The listing builds one solid part. Answer for the finished solid, in the listing's coordinates (mm). Face numbers are marked on the shaded views. A direction names the side the tool comes from. Coordinates: 2 decimals unless noted, no trailing zeros. Order: outer loops, then holes, each group sorted by start corner. A loop starts at its lowest first (then second) coordinate and runs counter-clockwise, first axis right, second up. Notation, with made-up numbers: (-20, 82.5) -> (33, 82.5) arc R18 cw to (33, 100.5) -> close; hole circle Ø11 at (72, 85). An arc over 180 degrees is marked (long way). Return JSON: item names as keys, results as strings.
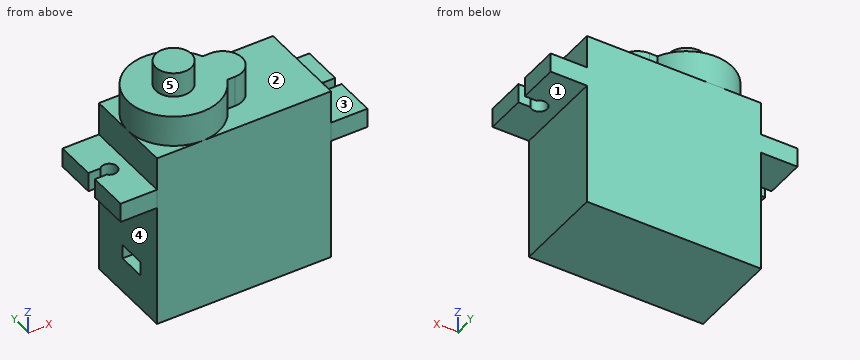
from build123d import *

# Parameters (mm, degrees)
CROQUIS1_W              = 22.5
CROQUIS1_H              = 11.8
SALIENTE_EXTRUIR1_DEPTH = 22.7
SALIENTE_EXTRUIR2_DEPTH = 2.5
SALIENTE_EXTRUIR3_DEPTH = 4
CROQUIS4_R              = 2.3
SALIENTE_EXTRUIR4_DEPTH = 3.2
CROQUIS5_W              = 1.844144091
CROQUIS5_H              = 3.6
CORTAR_EXTRUIR1_DEPTH   = 1.6


with BuildPart() as part:
    # Croquis1 → Saliente-Extruir1 (new body)
    with BuildSketch(Plane.XY):
        Rectangle(CROQUIS1_W, CROQUIS1_H)
    extrude(amount=SALIENTE_EXTRUIR1_DEPTH)

    # Croquis2 → Saliente-Extruir2 (add)
    with BuildSketch(Plane.XY.offset(15.9)):
        with BuildLine():
            Line((11.25, 5.9), (15.95, 5.9))
            Line((15.95, 5.9), (15.95, 0.647985587))
            Line((15.95, 0.647985587), (14.411652597, 0.647985587))
            ThreePointArc((14.411652597, 0.647985587), (12.650003513, 0.00265078), (14.408206572, -0.652014413))
            Line((14.408206572, -0.652014413), (15.95, -0.652014413))
            Line((15.95, -0.652014413), (15.95, -5.904028826))
            Line((15.95, -5.904028826), (11.25, -5.904028826))
            Line((11.25, -5.904028826), (11.25, 5.9))
        make_face()
        with BuildLine():
            Line((-11.25, 5.9), (-15.95, 5.9))
            Line((-15.95, 5.9), (-15.95, 0.647985587))
            Line((-15.95, 0.647985587), (-14.411652597, 0.647985587))
            ThreePointArc((-14.411652597, 0.647985587), (-12.650003513, 0.00265078), (-14.408206572, -0.652014413))
            Line((-14.408206572, -0.652014413), (-15.95, -0.652014413))
            Line((-15.95, -0.652014413), (-15.95, -5.904028826))
            Line((-15.95, -5.904028826), (-11.25, -5.904028826))
            Line((-11.25, -5.904028826), (-11.25, 5.9))
        make_face()
    extrude(amount=SALIENTE_EXTRUIR2_DEPTH)

    # Croquis3 → Saliente-Extruir3 (add)
    with BuildSketch(Plane.XY.offset(22.7)):
        with BuildLine():
            Line((1.003159638, -2.50231492), (-0.006927846, -2.50231492))
            ThreePointArc((-0.006927846, -2.50231492), (-11.24999987, 0.001237918), (-0.005878262, 2.500072568))
            Line((-0.005878262, 2.500072568), (1.003159638, 2.500072568))
            ThreePointArc((1.003159638, 2.500072568), (3.504353382, -0.001121176), (1.003159638, -2.50231492))
        make_face()
    extrude(amount=SALIENTE_EXTRUIR3_DEPTH)

    # Croquis4 → Saliente-Extruir4 (add)
    with BuildSketch(Plane.XY.offset(26.7)):
        with Locations((-5.35, 0)):
            Circle(CROQUIS4_R)
    extrude(amount=SALIENTE_EXTRUIR4_DEPTH)

    # Croquis5 → Cortar-Extruir1 (cut, symmetric)
    with BuildSketch(Plane.ZY.offset(11.25)):
        with Locations((5.422072046, -0.7)):
            Rectangle(CROQUIS5_W, CROQUIS5_H)
    extrude(amount=CORTAR_EXTRUIR1_DEPTH, both=True, mode=Mode.SUBTRACT)


solid = part.part
1. Consider line 1 (Y direction, x = -13.65, z = 17.4); line 2 (Y direction, x = 8.5, z = 10.75); line 3 (Z direction, x = -11.5, y = 1.75). Determine where each line is inside the solid, lowest interval first. Write a range as from..to.
Answer block:
{"line 1": "y = -5.9..-1, 1..5.9", "line 2": "y = -5.9..5.9", "line 3": "z = 15.9..18.4"}
2. The part is cut by section C-C on z = 7.5. Give the vertices of the cut face in (x, y), and give its area (4 significant figures).
Answer block:
{"outline": "(-11.25, -5.9) -> (11.25, -5.9) -> (11.25, 5.9) -> (-11.25, 5.9) -> close", "area": "265.5 mm2"}
3. The part is cut by section A-A on x = -13.65. Give the vertices of the cut face in (y, z), and give its area (3 significant figures).
Answer block:
{"outline": "(-5.9, 15.9) -> (-1, 15.9) -> (-1, 18.4) -> (-5.9, 18.4) -> close; (1, 15.9) -> (5.9, 15.9) -> (5.9, 18.4) -> (1, 18.4) -> close", "area": "24.5 mm2"}
4. Each of these flat-tipped pins is pushed along its axis until it touches: pin 1 Ø2.5 at (x, y) = (-13.5, -2.5) entering from +Z; pin 2 Ø3.5 at (y, z) = (0, 11.5) entering from -X; pin 3 Ø5 at (x, y) = (-7.5, -4.5) entering from +Z. Where does it stop, or does it pass through?
Answer block:
{"pin 1": "stops at z = 18.4", "pin 2": "stops at x = -11.25", "pin 3": "stops at z = 26.7"}
5. The part is cut by section D-D on x = -6.5. Give the vertices of the cut face in (y, z).
Answer block:
{"outline": "(-5.9, 0) -> (5.9, 0) -> (5.9, 22.7) -> (5.79, 22.7) -> (5.79, 26.7) -> (1.99, 26.7) -> (1.99, 29.9) -> (-1.99, 29.9) -> (-1.99, 26.7) -> (-5.79, 26.7) -> (-5.79, 22.7) -> (-5.9, 22.7) -> close"}
6. For the marked faces 1, 2, 3, 4 and 5, determine the directions among +Z, -Z, +X, -X, +Y, -Y from which every point of the face is accessible in a straight line to the end or side of a thin tool.
Answer block:
{"face 1": "-Z, +X, +Y, -Y", "face 2": "+Z, +X", "face 3": "+Z, +X, +Y, -Y", "face 4": "-Z, -X, +Y, -Y", "face 5": "+Z"}
7. The part is cut by section B-B on y = -4. Give the vertices of the cut face in (x, z), and give its area (3 significant figures).
Answer block:
{"outline": "(-15.95, 15.9) -> (-11.25, 15.9) -> (-11.25, 0) -> (11.25, 0) -> (11.25, 15.9) -> (15.95, 15.9) -> (15.95, 18.4) -> (11.25, 18.4) -> (11.25, 22.7) -> (-1.01, 22.7) -> (-1.01, 26.7) -> (-9.69, 26.7) -> (-9.69, 22.7) -> (-11.25, 22.7) -> (-11.25, 18.4) -> (-15.95, 18.4) -> close", "area": "569 mm2"}
